Part model, mm, in its own coordinate system. Round coordinates to 2 decimals unless told otherwise and drop trailing zeros. Loops run counter-clockwise (first coordinate to the right, second up) from the corner with the lowest first, then second, coordinate; pieces in that order, holes last. Notation, with made-up numbers: (14.5, 43) - (37.5, 43) arc R18 ccw to (37.5, 69) - close; hole circle Ø4 at (20.25, 69). An arc over 180 degrees is marked (long way). Write each question's results on one line, items separated by ' | '. Start each with the question number.
(1) Flat gauge pins, fed straight in: P1, Ø6, axis at x = -22, z = 33, coming from the +Y side; P2, Ø1.5, axis at x = -12.5, y = -1, coming from the +Z side; P3, Ø0.9, axis at x = 31.5, y = -1.5, coming from the +Z side; P4, Ø1.5, axis at y = -2, z = 3.5, coming from the -X side. Where does each tip first touch, or does it go through?
(2) Cut at C-C, the plane z = -29.5. List the corners of the cut face in (x, y), then the cut area to 3 significant figures.
(3) Drill centre lines: L1, parallel to X at y = -2.2, z = -33; L2, parallel to Z at x = -12.5, y = -2.3; L3, parallel to X at y = -2.05, z = 6. Where is each one in solid material? Low to high.
(4) Cut at B-B, the plane x = 11.5. List the corners of the cut face in (y, z), then the cut area to 3 significant figures.
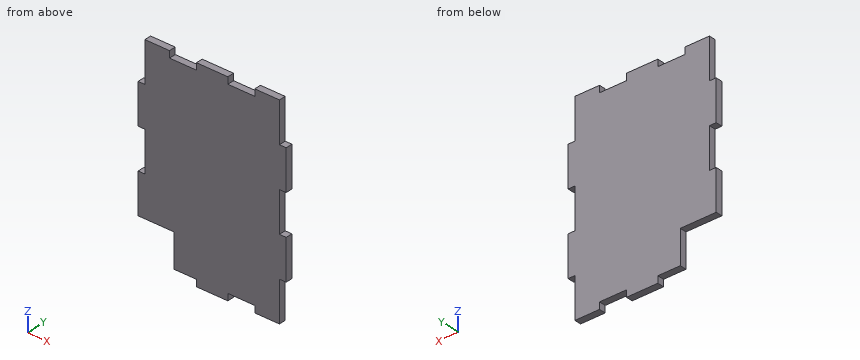
from build123d import *

# Parameters (mm, degrees)
F1_DEPTH = 3


with BuildPart() as f1:
    # F0 (on Front) → F1 (new body)
    with BuildSketch(Plane.XZ):
        Polygon((-19, 45), (-30, 45), (-30, 27), (-33, 27), (-33, 9), (-30, 9), (-30, -9), (-33, -9), (-33, -27), (-30, -27), (-17, -27), (-17, -42), (-7, -42), (-7, -45), (7, -45), (7, -42), (19, -42), (19, -45), (30, -45), (30, -27), (33, -27), (33, -9), (30, -9), (30, 9), (33, 9), (33, 27), (30, 27), (30, 45), (19, 45), (19, 42), (7, 42), (7, 45), (-7, 45), (-7, 42), (-19, 42), align=None)
    extrude(amount=F1_DEPTH)


solid = f1.part
A:
1) P1: y = 0 | P2: z = 42 | P3: z = 27 | P4: x = -30
2) outline: (-17, -3) - (30, -3) - (30, 0) - (-17, 0) - close | area: 141 mm2
3) L1: -17 to 30 | L2: -42 to 42 | L3: -30 to 30
4) outline: (-3, -42) - (0, -42) - (0, 42) - (-3, 42) - close | area: 252 mm2
